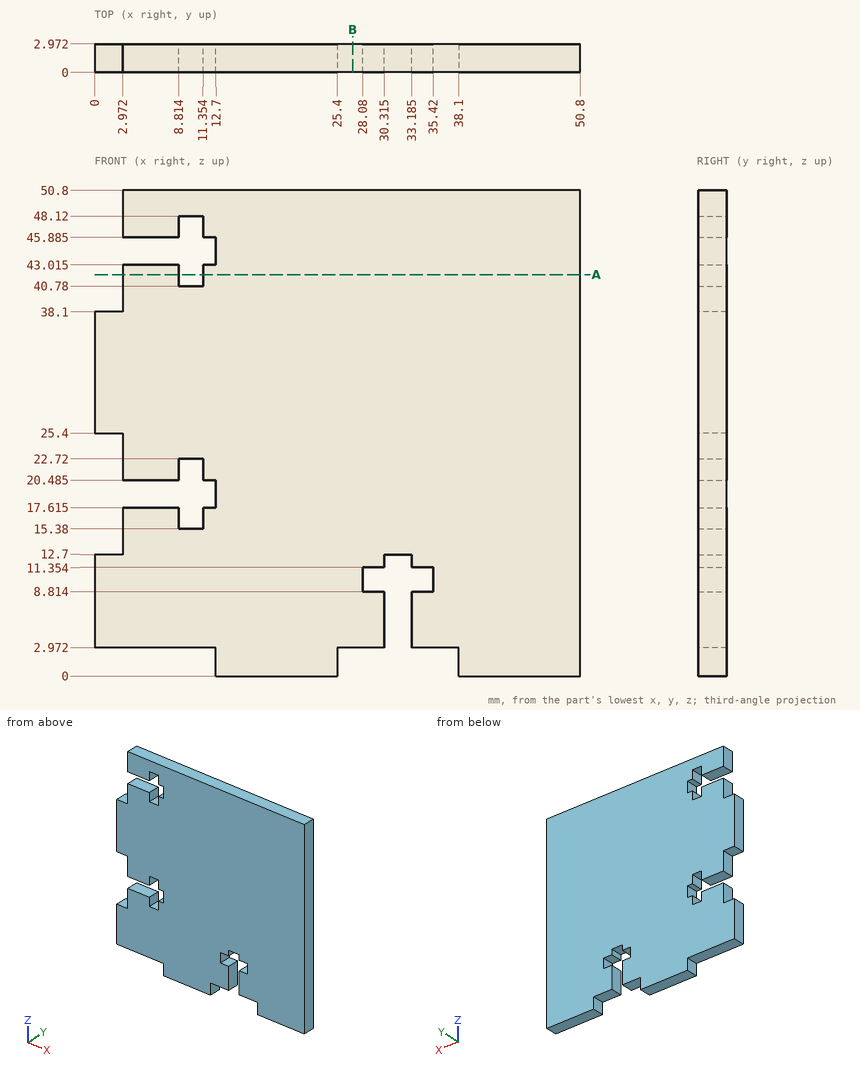
Design review of the part shown in the three views and the two pictorial views. Dimensions are in mm from the part's minimum x, y and z. Round coordinates to 2 decimals unless told otherwise and drop trailing zeros. Loops run counter-clockwise (first coordinate to the right, second up) from the corner with the lowest first, then second, coordinate; pieces in that order, holes last. Notation, with made-up numbers: M 69,28 L 125,28 A22 cw 125,48 Z; hole C 24,-19.5 d3. An arc over 180 degrees is marked long. Put each result on its own line as item: value.
Q1. Consider section B-B, the plane x = 27. Give the boundary of the cut face in (y, z), then the cut area to 3 significant figures.
Result set:
outline: M 0,2.97 L 2.97,2.97 L 2.97,50.8 L 0,50.8 Z
area: 142 mm²
Q2. To check wall thickness, follow L1, parallel to Z at x = 11.5, y = 1.05 (1 decimal); L2, parallel to Z at x = 29, y = 1.1. State the ranges of each line that lie inside material, in increasing order.
Result set:
L1: z = 3 to 17.6, 20.5 to 43, 45.9 to 50.8
L2: z = 2.97 to 8.81, 11.35 to 50.8
Q3. For pin 1 (1.4 mm diameter, centred on x = 31.5, y = 1, fed in from -Z); pin 2 (0.8 mm diameter, centred on x = 10, y = 1, fed in from -Z); pin 3 (0.9 mm diameter, centred on y = 1, z = 41, fed in from -X), all flat-tipped, find the tip position at first contact; note any pin that passes through.
Result set:
pin 1: stops at z = 12.7
pin 2: stops at z = 2.97
pin 3: stops at x = 2.97
Q4. Consider section A-A, the plane z = 42. Give the boundary of the cut face in (x, y).
Result set:
outline: M 2.97,0 L 8.81,0 L 8.81,2.97 L 2.97,2.97 Z; M 11.35,0 L 50.8,0 L 50.8,2.97 L 11.35,2.97 Z
